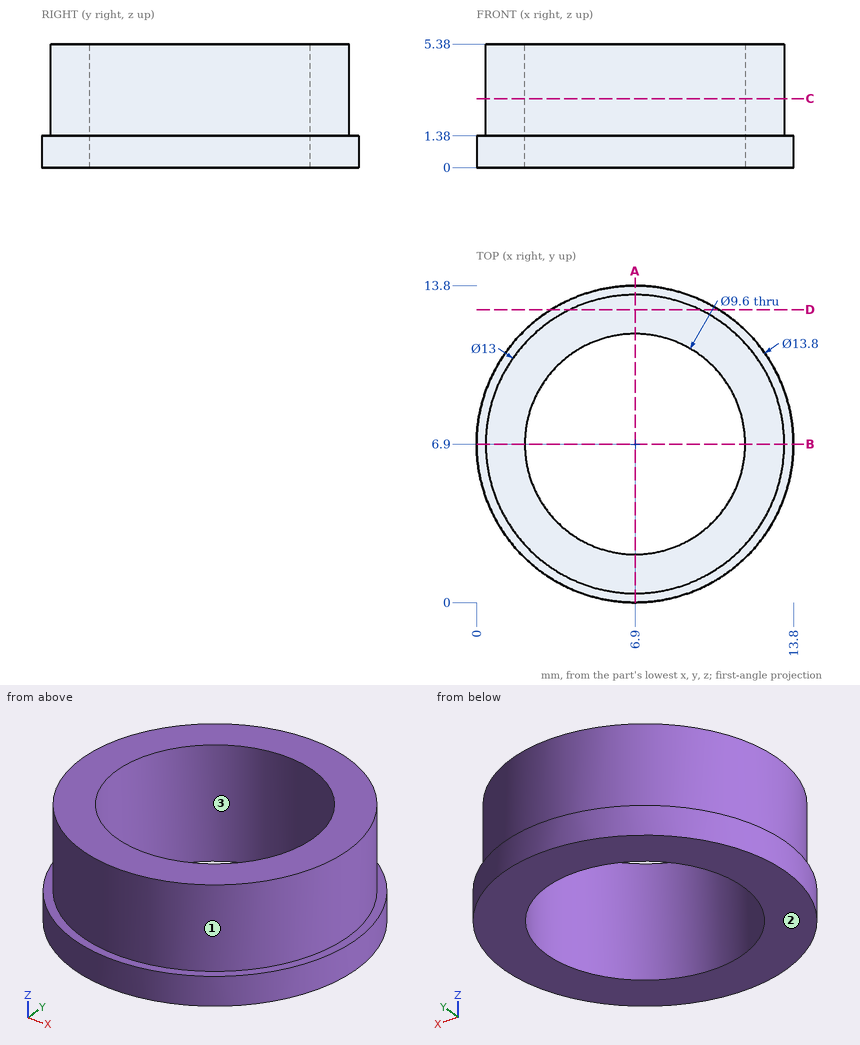
Check sheet for the drawn part. Datum: minimum x, y, z corner. Units: mm. Give positions to 0.01 mm unless a question says otherwise; leave off trailing zeros. Order: outer loops, then holes, each group sorted by start corner. A loop starts at its lowest first (then second) coordinate and runs counter-clockwise, first axis right, second up. Notation, with made-up numbers: (75, -7) -> (82, -7) arc R31 cw to (82, 25) -> close; hole circle Ø5 at (21, -33.5). An arc over 180 degrees is marked (long way). Return JSON: item names as keys, results as strings.
1. Go/stop test with flat-tipped pins: P1, Ø1, axis at y = 6, z = 0.5, coming from the -X side; P2, Ø3, axis at x = 8.5, z = 3.5, coming from the +Y side; P3, Ø1.5, axis at y = 7, z = 2.5, coming from the -X side. Record where each tip stops, or that it passes through.
From the geometry:
{"P1": "x = 0.01", "P2": "y = 13.4", "P3": "x = 0.4"}
2. Mould release check, pull along X, two halves, no side actions. Record for the marked faces 1, 2 and 3: +X half, -X half, draft (parallel to the pull), parting line (faces both ways), or undercut.
From the geometry:
{"face 1": "parting line", "face 2": "draft", "face 3": "undercut"}
3. Cross-section at A-A, the plane x = 6.9. Record the cut outline in (y, z).
From the geometry:
{"outline": "(0, 0) -> (2.1, 0) -> (2.1, 5.38) -> (0.4, 5.38) -> (0.4, 1.38) -> (0, 1.38) -> close; (11.7, 0) -> (13.8, 0) -> (13.8, 1.38) -> (13.4, 1.38) -> (13.4, 5.38) -> (11.7, 5.38) -> close"}
4. Cross-section at D-D, the plane y = 12.75. Record the cut outline in (x, z).
From the geometry:
{"outline": "(3.24, 0) -> (10.56, 0) -> (10.56, 1.38) -> (9.73, 1.38) -> (9.73, 5.38) -> (4.07, 5.38) -> (4.07, 1.38) -> (3.24, 1.38) -> close"}
5. Material ranges on probe 1 along Y at (x, z) = (6.9, 4); probe 2 along X at (y, z) = (3.5, 2.75); probe 3 along Y at (x, z) = (2.5, 2.7), recorded low to high. Write a range as [from, to].
From the geometry:
{"probe 1": "[0.4, 2.1], [11.7, 13.4]", "probe 2": "[1.36, 3.51], [10.29, 12.44]", "probe 3": "[2.12, 4.98], [8.82, 11.68]"}
6. Cross-section at C-C, the plane z = 3. Record the cut outline in (x, y).
From the geometry:
{"outline": "circle Ø13 at (6.9, 6.9); hole circle Ø9.6 at (6.9, 6.9)"}
